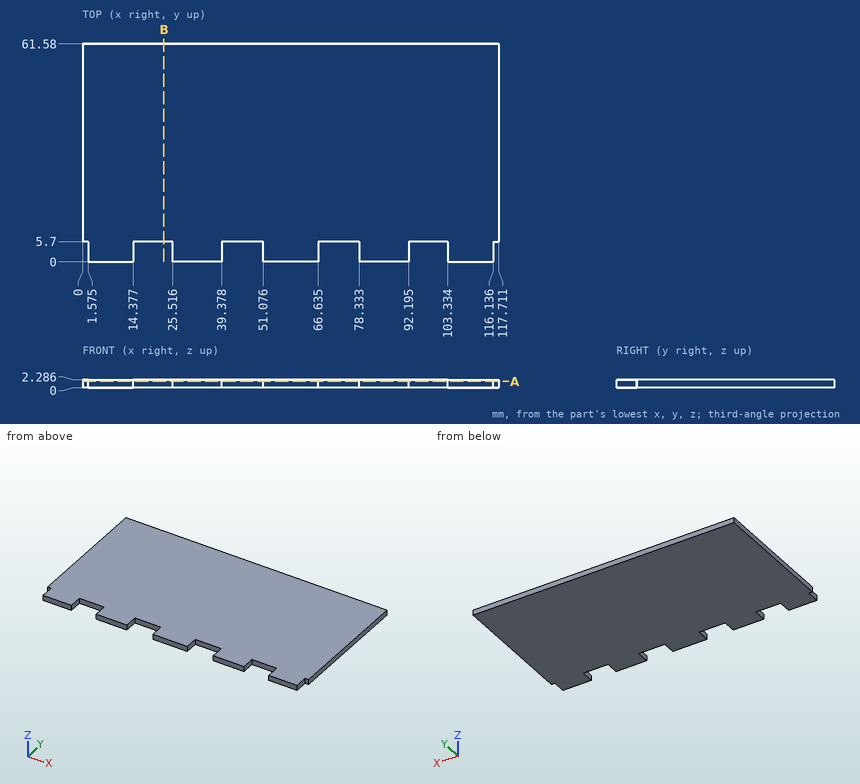
Geometry: see drawing. Coordinates: mm, zero at the bounding-box minimum. Round coordinates to 2 decimals unless told otherwise and drop trailing zeros. Loops run counter-clockwise (first coordinate to the right, second up) from the corner with the lowest first, then second, coordinate; pieces in that order, holes last. Notation, with made-up numbers: M 86,66 L 143,66 A27 ccw 143,100 Z; hole C 18.5,48.25 d2. An arc over 180 degrees is marked long. Use a Markdown table: item, result. Add a question column.
1. Line query: line 1 (X direction, y = 4, z = 1.1) (1 decimal); line 2 (Y direction, x = 17.5, z = 0.95). Output: solid intervals per line, ascending.
2. Section query A-A on z = 1.85. Return the cut outline in (x, y) (1 decimal).
3. Contact query for flat-ended pins moving along their axis: P1, Ø0.7, axis at y = 1.5, z = 1, coming from the +X side; P2, Ø1.1, axis at y = 3.5, z = 1.5, coming from the -X side (1 decimal); P3, Ø0.5, axis at x = 0.5, z = 1.5, coming from the -Y side. Output: stop coordinate, or through.
4. Section query B-B on x = 23. Return the cut outline in (y, z) (1 decimal), then the cut area to 3 significant figures.
Reported:
| question | item | result |
|---|---|---|
| 1 | line 1 | x = 1.6 to 14.4, 25.5 to 39.4, 51.1 to 66.6, 78.3 to 92.2, 103.3 to 116.1 |
| 1 | line 2 | y = 5.7 to 61.58 |
| 2 | outline | M 0,5.7 L 1.6,5.7 L 1.6,0 L 14.4,0 L 14.4,5.7 L 25.5,5.7 L 25.5,0 L 39.4,0 L 39.4,5.7 L 51.1,5.7 L 51.1,0 L 66.6,0 L 66.6,5.7 L 78.3,5.7 L 78.3,0 L 92.2,0 L 92.2,5.7 L 103.3,5.7 L 103.3,0 L 116.1,0 L 116.1,5.7 L 117.7,5.7 L 117.7,61.6 L 0,61.6 Z |
| 3 | P1 | stops at x = 116.14 |
| 3 | P2 | stops at x = 1.6 |
| 3 | P3 | stops at y = 5.7 |
| 4 | outline | M 5.7,0 L 61.6,0 L 61.6,2.3 L 5.7,2.3 Z |
| 4 | area | 128 mm² |
